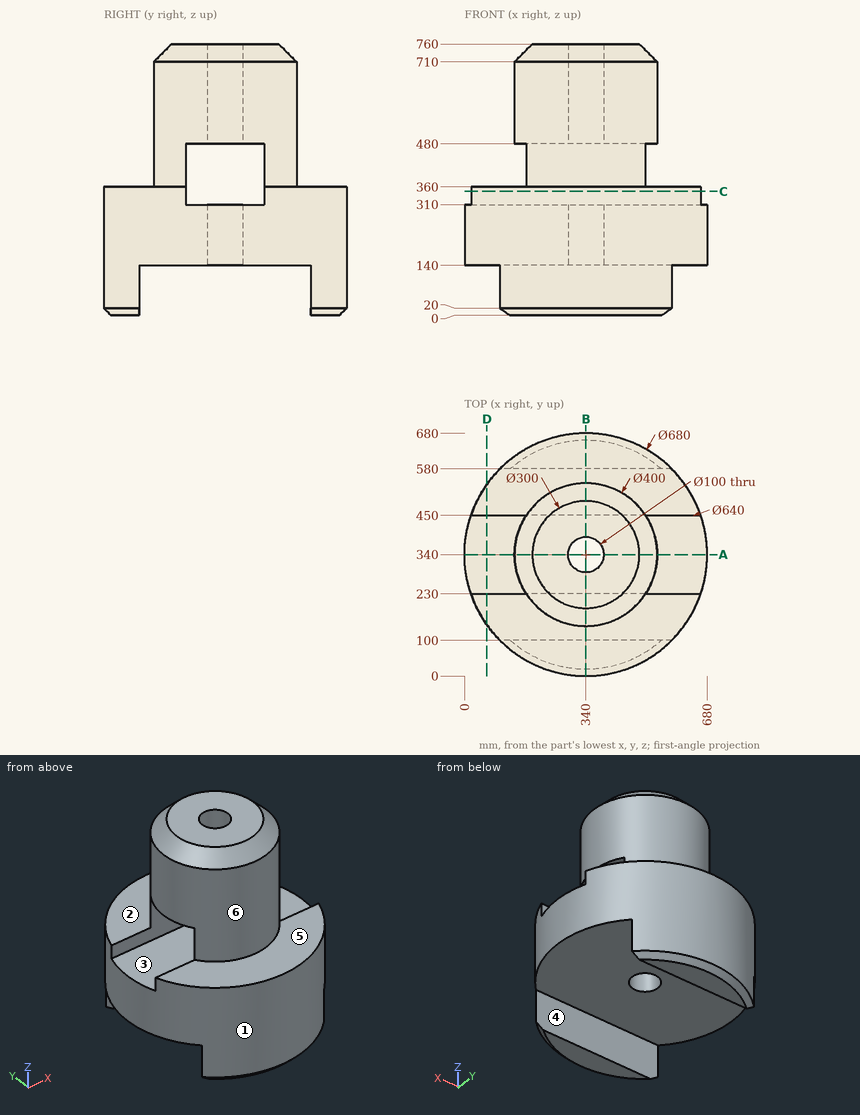
The figure shows three views and two pictorial views of one solid part (mm, origin at its lowest corner). Answer the questions. A direction names the side the tool comes from. Coordinates: 2 decimals unless noted, no trailing zeros. Loops run counter-clockwise (first coordinate to the right, second up) from the corner with the lowest first, then second, coordinate; pieces in that order, holes last. Notation, with made-up numbers: (11, -24.75) - (27, -24.75) arc R20 cw to (27, -5.75) - close; hole circle Ø1 at (51, 13.5). An arc over 180 degrees is marked (long way). Answer in a Markdown table with one row per item.
Q1. Find section A-A on y = 340. Write down the section's boundary in (x, z), plus the area to 3 significant figures.
Here are the results:
| item | result |
|---|---|
| outline | (0, 140) - (290, 140) - (290, 310) - (0, 310) - close; (140, 480) - (290, 480) - (290, 760) - (190, 760) - (140, 710) - close; (390, 140) - (680, 140) - (680, 310) - (390, 310) - close; (390, 480) - (540, 480) - (540, 710) - (490, 760) - (390, 760) - close |
| area | 180,000 mm^2 |
Q2. Given P1, Ø8, axis at x = 79.5, y = 140.5, coming from the -Z side; P2, Ø4, axis at x = 490, z = 143, coming from the -Y side; P3, Ø6, axis at y = 578.5, z = 247, coming from the -X side, each flat-ended and moving along its own axis, determine where each tip first touches the part or whether it passes through.
Here are the results:
| item | result |
|---|---|
| P1 | stops at z = 140 |
| P2 | stops at y = 33.9 |
| P3 | stops at x = 94.77 |
Q3. For the marked faces 4, 5 and 6, determine the directions among +Z, -Z, +X, -X, +Y, -Y from which every point of the face is accessible in a straight line to the end or side of a thin tool.
Here are the results:
| item | result |
|---|---|
| face 4 | -Z, +X, -X |
| face 5 | +Z, -Y |
| face 6 | +Z |
Q4. Find section C-C on z = 347. Write down the section's boundary in (x, y).
Here are the results:
| item | result |
|---|---|
| outline | (18.29, 230) arc R340 ccw to (661.71, 230) - close; (18.29, 450) - (661.71, 450) arc R340 ccw to start |
Q5. The mould has two halves that part along Y. Classify the marked faces 1, 2 and 3: pulls with the +Y half, pulls with the -Y half, needs draft (parallel to the pull), parting line crosses it, or undercut.
Here are the results:
| item | result |
|---|---|
| face 1 | parting line crosses it |
| face 2 | needs draft |
| face 3 | undercut |
Q6. Straight lines are drawn through the part: line 1 along Z through (x, y) = (406.5, 370); line 2 along Y through (x, z) = (340, 188); line 3 along Y through (x, z) = (340, 692.5). For each, find the intervals that lie inside material, in ascending order. Write a range as [from, to].
Here are the results:
| item | result |
|---|---|
| line 1 | z = [140, 310], [480, 760] |
| line 2 | y = [0, 290], [390, 680] |
| line 3 | y = [140, 290], [390, 540] |
Q7. Find section D-D on x = 62.5. Write down the section's boundary in (y, z), plus the area to 3 significant figures.
Here are the results:
| item | result |
|---|---|
| outline | (143.55, 140) - (536.45, 140) - (536.45, 360) - (450, 360) - (450, 310) - (230, 310) - (230, 360) - (143.55, 360) - close |
| area | 75,400 mm^2 |
Q8. Find section B-B on x = 340. Write down the section's boundary in (y, z).
Here are the results:
| item | result |
|---|---|
| outline | (0, 20) - (20, 0) - (100, 0) - (100, 140) - (290, 140) - (290, 310) - (230, 310) - (230, 480) - (290, 480) - (290, 760) - (190, 760) - (140, 710) - (140, 360) - (0, 360) - close; (390, 140) - (580, 140) - (580, 0) - (660, 0) - (680, 20) - (680, 360) - (540, 360) - (540, 710) - (490, 760) - (390, 760) - (390, 480) - (450, 480) - (450, 310) - (390, 310) - close |
